Verification items for the finished model (mm, model axes). Face numbers are marked on the shaded views. A direction names the side the tool comes from. Coordinates: 2 decimals unless noted, no trailing zeros. Write each loop counter-clockwise with the first axis right and the second up, starting at its lowest first coordinate (ties: lowest second). Pieces come first, ordered by that corner, then holes. Notation, with made-up numbers: M -39,60 L 17,60 A22 cw 17,86 Z; hole C 65,1.5 d3. An arc over 180 degrees is marked long. Answer in a Markdown table with one row per item.
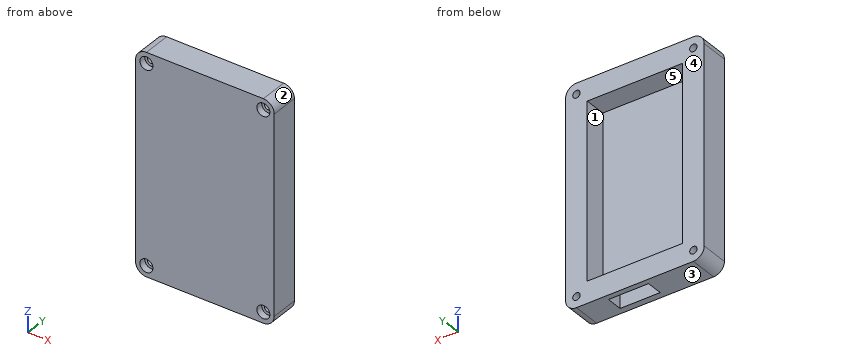
Autodesk Fusion 360 part; units mm, degrees
sketch "Sketch1" plane through (0, 0, 0) normal (0, 1, 0) x (1, 0, 0)
  line L0 (22, 40.5) -> (-22, 40.5)
  line L1 (-22, 40.5) -> (-22, -40.5)
  line L2 (-22, -40.5) -> (22, -40.5)
  line L3 (22, -40.5) -> (22, 40.5)
  line L4 (22, 40.5) -> (-22, -40.5) construction
  line L5 (-22, 40.5) -> (22, -40.5) construction
  line L6 (32, 50.5) -> (-32, 50.5)
  line L7 (-32, 50.5) -> (-32, -50.5)
  line L8 (-32, -50.5) -> (32, -50.5)
  line L9 (32, -50.5) -> (32, 50.5)
  line L10 (32, 50.5) -> (-32, -50.5) construction
  line L11 (-32, 50.5) -> (32, -50.5) construction
  line L12 (-32, 50.5) -> (-27, 50.5)
  line L13 (-32, 45.5) -> (-32, 50.5)
  circle A0 centre (-27, 45.5) radius 1.7
  circle A1 centre (-27, 45.5) radius 3
  line L14 (32, 50.5) -> (27, 50.5)
  line L15 (32, 45.5) -> (32, 50.5)
  circle A2 centre (27, 45.5) radius 1.7
  circle A3 centre (27, 45.5) radius 3
  line L16 (32, -50.5) -> (27, -50.5)
  line L17 (32, -45.5) -> (32, -50.5)
  circle A4 centre (27, -45.5) radius 1.7
  circle A5 centre (27, -45.5) radius 3
  line L18 (-32, -50.5) -> (-27, -50.5)
  line L19 (-32, -45.5) -> (-32, -50.5)
  circle A6 centre (-27, -45.5) radius 1.7
  circle A7 centre (-27, -45.5) radius 3
  dimension "d1" = 44
  dimension "d2" = 81
  dimension "d3" = 64
  dimension "d4" = 101
  dimension "d5" = 5
  dimension "d6" = 5
  dimension "d7" = 3.4
  dimension "d8" = 6
  dimension "d9" = 5
  dimension "d10" = 5
  dimension "d11" = 3.4
  dimension "d12" = 6
  dimension "d13" = 5
  dimension "d14" = 5
  dimension "d15" = 3.4
  dimension "d16" = 6
  dimension "d17" = 5
  dimension "d18" = 5
  dimension "d19" = 3.4
  dimension "d20" = 6
extrude "Extrude1" add sketch "Sketch1" along normal blind 9.9 from surface at 3.1 contours A1 | A3 | A5 | A7 makes body 1 at (29.9963, 9.7, 45.6495) makes body 2 at (-29.9963, 9.7, 45.6495) makes body 3 at (29.9963, 9.7, -45.3505) makes body 4 at (-29.9963, 9.7, -45.3505)
extrude "Extrude2" add sketch "Sketch1" along normal blind 13 contours L6 L7 L8 L9 L12 L13 L14 L15 L16 L17 L18 L19 bodies 1 2 3 4
extrude "Extrude3" add sketch "Sketch1" along normal blind 3 contours L0 L1 L2 L3 bodies 1
sketch "Sketch2" plane through (0, 3, 0) normal (0, 1, 0) x (-1, 0, 0)
  line L0 (-22, 40.5) -> (-22, -40.5)
  line L1 (-22, -40.5) -> (22, -40.5)
  line L2 (22, -40.5) -> (22, 40.5)
  line L3 (22, 40.5) -> (-22, 40.5)
  line L4 (-22, -40.5) -> (-32, -40.5)
  line L5 (-32, -40.5) -> (-32, -50.5)
  line L6 (-32, -50.5) -> (-22, -50.5)
  line L7 (-22, -50.5) -> (-22, -40.5)
  line L8 (-22, -50.5) -> (-14, -50.5)
  line L9 (-14, -50.5) -> (-14, -40.5)
  line L10 (-14, -40.5) -> (-22, -40.5)
  line L11 (-22, -40.5) -> (-22, -50.5)
  line L12 (-14, -50.5) -> (4.5, -50.5)
  line L13 (4.5, -50.5) -> (4.5, -40.5)
  line L14 (4.5, -40.5) -> (-14, -40.5)
  line L15 (-14, -40.5) -> (-14, -50.5)
  dimension "d28" = 10
  dimension "d29" = 10
  dimension "d30" = 8
  dimension "d31" = 10
  dimension "d32" = 18.5
  dimension "d33" = 10
extrude "Extrude4" cut sketch "Sketch2" along normal blind 7.5 contours L1 L9 L12 L13 L14 L15 bodies 1
fillet "Fillet1" radius 5 1 edges at (-32, 6.5, -50.5) on bodies 1
fillet "Fillet2" radius 5 1 edges at (32, 6.5, -50.5) on bodies 1
fillet "Fillet3" radius 5 1 edges at (32, 6.5, 50.5) on bodies 1
fillet "Fillet4" radius 5 1 edges at (-32, 6.5, 50.5) on bodies 1
sketch "Sketch3" plane through (0, 3, 0) normal (0, 1, 0) x (-1, 0, 0)
  line L0 (-22, 40.5) -> (-22, -40.5)
  line L1 (-22, -40.5) -> (-14, -40.5)
  line L2 (-14, -40.5) -> (-14, -50.5)
  line L3 (-14, -50.5) -> (4.5, -50.5)
  line L4 (4.5, -50.5) -> (4.5, -40.5)
  line L5 (4.5, -40.5) -> (22, -40.5)
  line L6 (22, -40.5) -> (22, 40.5)
  line L7 (22, 40.5) -> (-22, 40.5)
1) Sectioned sample at A-A (x = 6). Record the cut outline in (y, z), then the cut area to 3 significant figures.
Response values:
| item | result |
|---|---|
| outline | M 0,-50.5 L 3,-50.5 L 3,40.5 L 13,40.5 L 13,50.5 L 0,50.5 Z; M 10.5,-50.5 L 13,-50.5 L 13,-40.5 L 10.5,-40.5 Z |
| area | 428 mm² |
2) Sectioned sample at D-D (x = 16). Record the cut outline in (y, z).
Response values:
| item | result |
|---|---|
| outline | M 0,-50.5 L 13,-50.5 L 13,-40.5 L 3,-40.5 L 3,40.5 L 13,40.5 L 13,50.5 L 0,50.5 Z |
3) Release check for a two-part mould opening along Z. For the marked faces 3, 4 and 5 record: +Z half, -Z half, draft (parallel to the pull), parting line (faces both ways), or undercut.
Response values:
| item | result |
|---|---|
| face 3 | -Z half |
| face 4 | draft |
| face 5 | undercut |
4) Depth check by flat-ended pin: pin 1 (8 mm diameter, centred on x = -4, z = 34, fed in from +Y); pin 2 (9.5 mm diameter, centred on x = -27, z = 45.5, fed in from -Y); pin 3 (4.5 mm diameter, centred on x = -27, z = 45.5, fed in from -Y). Enter the tip coordinate at first touch or a pass-through.
Response values:
| item | result |
|---|---|
| pin 1 | stops at y = 3 |
| pin 2 | stops at y = 0 |
| pin 3 | stops at y = 3.1 |
5) Tool access check on the marked faces 1 and 2. Record the directions out of +Z, -Z, +X, -X, +Y, -Y that give a thin tool (end or side, any length) a straight path to the whole face; none if there is none.
Response values:
| item | result |
|---|---|
| face 1 | +Y |
| face 2 | +Z, +X, +Y, -Y |
6) Sectioned sample at C-C (y = 6). Record the cut outline in (x, z).
Response values:
| item | result |
|---|---|
| outline | M -32,-45.5 A5 ccw -27,-50.5 L -4.5,-50.5 L -4.5,-40.5 L -22,-40.5 L -22,40.5 L 22,40.5 L 22,-40.5 L 14,-40.5 L 14,-50.5 L 27,-50.5 A5 ccw 32,-45.5 L 32,45.5 A5 ccw 27,50.5 L -27,50.5 A5 ccw -32,45.5 Z; hole C -27,-45.5 d3.4; hole C -27,45.5 d3.4; hole C 27,-45.5 d3.4; hole C 27,45.5 d3.4 |
7) Thickness scan on L1, parallel to X at y = 7, z = 45.5; L2, parallel to Z at x = 27, y = 9; L3, parallel to Z at x = 27, y = 2.4. Record the ranges inside material, lowest first. Write a range as [from, to].
Response values:
| item | result |
|---|---|
| L1 | x = [-32, -28.7], [-25.3, 25.3], [28.7, 32] |
| L2 | z = [-50.5, -47.2], [-43.8, 43.8], [47.2, 50.5] |
| L3 | z = [-50.5, -48.5], [-42.5, 42.5], [48.5, 50.5] |
8) Sectioned sample at B-B (z = 37.5). Record the cut outline in (x, y).
Response values:
| item | result |
|---|---|
| outline | M -32,0 L 32,0 L 32,13 L 22,13 L 22,3 L -22,3 L -22,13 L -32,13 Z |
